Work out the finished part from the listing and answer in its coordinate system (mm). Face numbers are marked on the shaded views. A direction names the side the tool comes from. Give positions to 0.01 mm unless a question says otherwise; leave off trailing zeros. Loops run counter-clockwise (first coordinate to the right, second up) from the corner with the lowest first, then second, coordinate; pieces in that order, holes last. Notation, with made-up numbers: (74, 16.5) - (104, 16.5) arc R20 ccw to (104, 31.5) - close; hole circle Ø10 at (-1.75, -36). An arc over 180 degrees is marked (long way). One line per question, with ' | ' between items. Start each with the question number.
1. Find the intervals of material crossed by line 1 (Z direction, x = -7, y = 8.25); line 2 (Z direction, x = 7, y = 8.5); line 3 (Y direction, x = -20.4, z = 0), in increasing order.
2. Section B-B (y = 8.5) is taken. Determine the outline of the cut face in (x, z).
3. Each of these flat-tipped pins is pushed along its axis until it touches: pin 1 (3.5 mm diameter, centred on y = 8, z = 0, fed in from -X); pin 2 (4.5 mm diameter, centred on x = 0, y = -3, fed in from -Z); pin 3 (4 mm diameter, centred on y = -3, z = 0, fed in from +X). Where does it stop, or does it pass through?
4. For a pull along Z with two mould halves and no side action, classify the marked faces 4, 5 and 6 as released by +Z, released by -Z, zero draft, split by the parting line, or undercut.
5. Section A-A (y = -3) is taken. Give the number of separate pieces and of enclosed holes in the cut face, plus the area to 3 significant figures.
6. Which of the six approach directions +Z, -Z, +X, -X, +Y, -Y give full straight-line access (tool end or side, diameter ignored) to the marked faces 1, 2 and 3?
from build123d import *

# Parameters (mm, degrees)
SKETCH_1_R                = 19
SKETCH_1_R_2              = 1.45
SKETCH_1_R_3              = 2
EXTRUDE_1_DEPTH           = 12
SKETCH_2_R                = 1.45
SKETCH_2_R_2              = 2
EXTRUDE_2_DEPTH           = 7
SKETCH_3_R                = 1.45
CUT_EXTRUDE_1_DEPTH       = 48.5
SKETCH_4_R                = 1.45
CUT_EXTRUDE_2_DEPTH       = 48.5
SKETCH_5_R                = 1.45
CUT_EXTRUDE_3_DEPTH       = 39
SKETCH_8_R                = 24
CUT_EXTRUDE_6_DEPTH       = 5
SKETCH_10_R               = 24.25
EXTRUDE_3_DEPTH           = 3
SKETCH_11_R               = 21.9
EXTRUDE_4_DEPTH           = 18
CUT_EXTRUDE_7_DEPTH       = 18
SKETCH_13_R               = 1.45
CUT_EXTRUDE_8_DEPTH       = 43.25
CUT_EXTRUDE_8_DEPTH_BACK  = 7.25
SKETCH_14_R               = 1.45
CUT_EXTRUDE_9_DEPTH       = 53.294678888
CUT_EXTRUDE_9_DEPTH_BACK  = 17.294678888
SKETCH_15_R               = 1.45
CUT_EXTRUDE_10_DEPTH      = 43.25
CUT_EXTRUDE_10_DEPTH_BACK = 7.25
SKETCH_16_R               = 1.5
CUT_EXTRUDE_11_DEPTH      = 53.294678888
CUT_EXTRUDE_11_DEPTH_BACK = 17.294678888
FILLET_1_R                = 0.5
FILLET_2_R                = 2
SKETCH_17_R               = 1.45
SKETCH_17_R_2             = 2
SKETCH_17_R_3             = 2.272593427
EXTRUDE_5_DEPTH           = 9


with BuildPart() as part:
    # 草图1 → 凸台-拉伸1 (new body)
    with BuildSketch(Plane(origin=(0, 0, 0), x_dir=(1, 0, 0), z_dir=(0, 1, 0))):
        Circle(SKETCH_1_R)
        with Locations((0, 13.5)):
            Circle(SKETCH_1_R_2, mode=Mode.SUBTRACT)
        with Locations((-11.691342951, -6.75)):
            Circle(SKETCH_1_R_2, mode=Mode.SUBTRACT)
        with Locations((11.691342951, -6.75)):
            Circle(SKETCH_1_R_2, mode=Mode.SUBTRACT)
        with Locations((-10.522208656, 6.075)):
            Circle(SKETCH_1_R_3, mode=Mode.SUBTRACT)
        with Locations((0, -12.15)):
            Circle(SKETCH_1_R_3, mode=Mode.SUBTRACT)
        with Locations((10.522208656, 6.075)):
            Circle(SKETCH_1_R_3, mode=Mode.SUBTRACT)
    extrude(amount=EXTRUDE_1_DEPTH)

    # 草图2 → 凸台-拉伸2 (add)
    with BuildSketch(Plane(origin=(0, 12, 0), x_dir=(1, 0, 0), z_dir=(0, 1, 0))):
        Polygon((0, 21.939310229), (-19, 10.969655115), (-19, -10.969655115), (0, -21.939310229), (19, -10.969655115), (19, 10.969655115), align=None)
        with Locations((0, 13.5)):
            Circle(SKETCH_2_R, mode=Mode.SUBTRACT)
        with Locations((-10.522208656, 6.075)):
            Circle(SKETCH_2_R_2, mode=Mode.SUBTRACT)
        with Locations((10.522208656, 6.075)):
            Circle(SKETCH_2_R_2, mode=Mode.SUBTRACT)
        with Locations((-11.691342951, -6.75)):
            Circle(SKETCH_2_R, mode=Mode.SUBTRACT)
        with Locations((0, -12.15)):
            Circle(SKETCH_2_R_2, mode=Mode.SUBTRACT)
        with Locations((11.691342951, -6.75)):
            Circle(SKETCH_2_R, mode=Mode.SUBTRACT)
    extrude(amount=-EXTRUDE_2_DEPTH)

    # 草图3 → 切除-拉伸1 (cut, through all)
    with BuildSketch(Plane(origin=(9.5, 0, 16.454482672), x_dir=(0.866025404, 0, -0.5), z_dir=(0.5, 0, 0.866025404))):
        with Locations((0, 8.5)):
            Circle(SKETCH_3_R)
    extrude(amount=-CUT_EXTRUDE_1_DEPTH, mode=Mode.SUBTRACT)

    # 草图4 → 切除-拉伸2 (cut, through all)
    with BuildSketch(Plane(origin=(-9.5, 0, 16.454482672), x_dir=(0.866025404, 0, 0.5), z_dir=(-0.5, 0, 0.866025404))):
        with Locations((0, 8.5)):
            Circle(SKETCH_4_R)
    extrude(amount=-CUT_EXTRUDE_2_DEPTH, mode=Mode.SUBTRACT)

    # 草图5 → 切除-拉伸3 (cut, through all)
    with BuildSketch(Plane.ZY.offset(19)):
        with Locations((0, 8.5)):
            Circle(SKETCH_5_R)
    extrude(amount=-CUT_EXTRUDE_3_DEPTH, mode=Mode.SUBTRACT)

    # 草图8 → 切除-拉伸6 (cut)
    with BuildSketch(Plane.XZ):
        Circle(SKETCH_8_R)
    extrude(amount=-CUT_EXTRUDE_6_DEPTH, mode=Mode.SUBTRACT)

    # 草图10 → 凸台-拉伸3 (add)
    with BuildSketch(Plane.XZ.offset(-5)):
        Circle(SKETCH_10_R)
    extrude(amount=EXTRUDE_3_DEPTH)

    # 草图11 → 凸台-拉伸4 (add)
    with BuildSketch(Plane.XZ.offset(-2)):
        Circle(SKETCH_11_R)
    extrude(amount=EXTRUDE_4_DEPTH)

    # 草图12 → 切除-拉伸7 (cut)
    with BuildSketch(Plane.XZ.offset(16)):
        with BuildLine():
            Line((-15.656854249, -9.798989873), (-9.798989873, -15.656854249))
            ThreePointArc((-9.798989873, -15.656854249), (-7.203603083, -17.39103626), (-4.142135624, -18))
            Line((-4.142135624, -18), (4.142135624, -18))
            ThreePointArc((4.142135624, -18), (7.203603083, -17.39103626), (9.798989873, -15.656854249))
            Line((9.798989873, -15.656854249), (15.656854249, -9.798989873))
            ThreePointArc((15.656854249, -9.798989873), (17.39103626, -7.203603083), (18, -4.142135624))
            Line((18, -4.142135624), (18, 4.142135624))
            ThreePointArc((18, 4.142135624), (17.39103626, 7.203603083), (15.656854249, 9.798989873))
            Line((15.656854249, 9.798989873), (9.798989873, 15.656854249))
            ThreePointArc((9.798989873, 15.656854249), (7.203603083, 17.39103626), (4.142135624, 18))
            Line((4.142135624, 18), (-4.142135624, 18))
            ThreePointArc((-4.142135624, 18), (-7.203603083, 17.39103626), (-9.798989873, 15.656854249))
            Line((-9.798989873, 15.656854249), (-15.656854249, 9.798989873))
            ThreePointArc((-15.656854249, 9.798989873), (-17.39103626, 7.203603083), (-18, 4.142135624))
            Line((-18, 4.142135624), (-18, -4.142135624))
            ThreePointArc((-18, -4.142135624), (-17.39103626, -7.203603083), (-15.656854249, -9.798989873))
        make_face()
    extrude(amount=-CUT_EXTRUDE_7_DEPTH, mode=Mode.SUBTRACT)

    # 草图13 → 切除-拉伸8 (cut, two sides)
    with BuildSketch(Plane.ZY.offset(-18)) as cut_extrude_8_sk:
        with Locations((0, -3)):
            Circle(SKETCH_13_R)
    extrude(amount=CUT_EXTRUDE_8_DEPTH, mode=Mode.SUBTRACT)
    extrude(cut_extrude_8_sk.sketch, amount=-CUT_EXTRUDE_8_DEPTH_BACK, mode=Mode.SUBTRACT)

    # 草图14 → 切除-拉伸9 (cut, two sides)
    with BuildSketch(Plane(origin=(12.727922061, 0, -12.727922061), x_dir=(0.707106781, 0, 0.707106781), z_dir=(-0.707106781, 0, 0.707106781))) as cut_extrude_9_sk:
        with Locations((0, -11)):
            Circle(SKETCH_14_R)
    extrude(amount=CUT_EXTRUDE_9_DEPTH, mode=Mode.SUBTRACT)
    extrude(cut_extrude_9_sk.sketch, amount=-CUT_EXTRUDE_9_DEPTH_BACK, mode=Mode.SUBTRACT)

    # 草图15 → 切除-拉伸10 (cut, two sides)
    with BuildSketch(Plane.XY.offset(-18)) as cut_extrude_10_sk:
        with Locations((0, -3)):
            Circle(SKETCH_15_R)
    extrude(amount=CUT_EXTRUDE_10_DEPTH, mode=Mode.SUBTRACT)
    extrude(cut_extrude_10_sk.sketch, amount=-CUT_EXTRUDE_10_DEPTH_BACK, mode=Mode.SUBTRACT)

    # 草图16 → 切除-拉伸11 (cut, two sides)
    with BuildSketch(Plane(origin=(-12.727922061, 0, -12.727922061), x_dir=(0.707106781, 0, -0.707106781), z_dir=(0.707106781, 0, 0.707106781))) as cut_extrude_11_sk:
        with Locations((0, -11)):
            Circle(SKETCH_16_R)
    extrude(amount=CUT_EXTRUDE_11_DEPTH, mode=Mode.SUBTRACT)
    extrude(cut_extrude_11_sk.sketch, amount=-CUT_EXTRUDE_11_DEPTH_BACK, mode=Mode.SUBTRACT)

    # 圆角1
    fillet_1_edges = [part.edges().sort_by_distance(p)[0] for p in [
        (-21.9, -16, 0),
        (-7.203603083, -16, 17.39103626),
        (-12.727922061, -16, 12.727922061),
        (-17.39103626, -16, 7.203603083),
        (-18, -16, 0),
        (-17.39103626, -16, -7.203603083),
        (-12.727922061, -16, -12.727922061),
        (-7.203603083, -16, -17.39103626),
        (0, -16, -18),
        (7.203603083, -16, -17.39103626),
        (12.727922061, -16, -12.727922061),
        (17.39103626, -16, -7.203603083),
        (18, -16, 0),
        (17.39103626, -16, 7.203603083),
        (12.727922061, -16, 12.727922061),
        (7.203603083, -16, 17.39103626),
        (0, -16, 18),
    ]]
    fillet(fillet_1_edges, radius=FILLET_1_R)

    # 圆角2
    fillet_2_edges = [part.edges().sort_by_distance(p)[0] for p in [
        (-7.203603083, 2, 17.39103626),
        (0, 2, 18),
        (7.203603083, 2, 17.39103626),
        (12.727922061, 2, 12.727922061),
        (17.39103626, 2, 7.203603083),
        (18, 2, 0),
        (17.39103626, 2, -7.203603083),
        (12.727922061, 2, -12.727922061),
        (7.203603083, 2, -17.39103626),
        (0, 2, -18),
        (-7.203603083, 2, -17.39103626),
        (-12.727922061, 2, -12.727922061),
        (-17.39103626, 2, -7.203603083),
        (-18, 2, 0),
        (-17.39103626, 2, 7.203603083),
        (-12.727922061, 2, 12.727922061),
    ]]
    fillet(fillet_2_edges, radius=FILLET_2_R)

    # 草图17 → 凸台-拉伸5 (add)
    with BuildSketch(Plane(origin=(0, 12, 0), x_dir=(1, 0, 0), z_dir=(0, 1, 0))):
        with Locations((0, 13.5)):
            Circle(SKETCH_17_R)
        with Locations((10.522208656, 6.075)):
            Circle(SKETCH_17_R_2)
        with Locations((11.691342951, -6.75)):
            Circle(SKETCH_17_R)
        with Locations((0, -12.15)):
            Circle(SKETCH_17_R_2)
        with Locations((-11.691342951, -6.75)):
            Circle(SKETCH_17_R)
        with Locations((-10.522208656, 6.075)):
            Circle(SKETCH_17_R_3)
    extrude(amount=-EXTRUDE_5_DEPTH)


solid = part.part
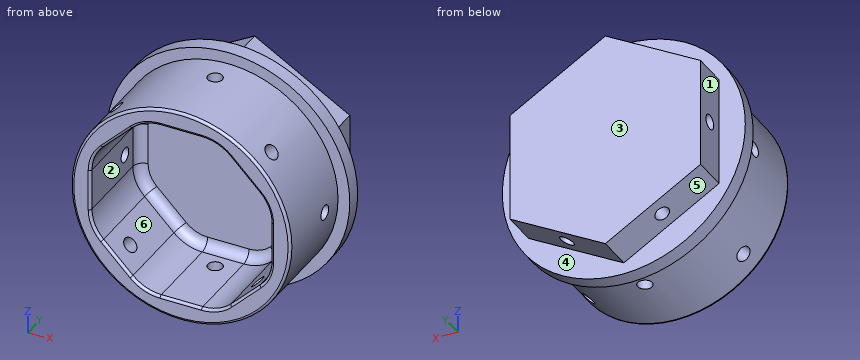
Conclusion:
1) line 1: -17.9 to -14.98, -9.27 to -1.43, 1.43 to 9.27, 14.98 to 17.9 | line 2: -17.9 to -15.02, -9.22 to -1.45, 1.45 to 9.22, 15.02 to 17.9 | line 3: -16 to -4.45, -1.55 to 5
2) outline: (-19, -10.97) - (-10.76, -15.73) - (-2.51, -1.45) - (-19, -1.45) - close; (-19, 1.45) - (-2.51, 1.45) - (-10.76, 15.73) - (-19, 10.97) - close; (-8.24, -17.18) - (0, -21.94) - (8.24, -17.18) - (0, -2.9) - close; (-8.24, 17.18) - (0, 2.9) - (8.24, 17.18) - (0, 21.94) - close; (2.51, -1.45) - (10.76, -15.73) - (19, -10.97) - (19, -1.45) - close; (2.51, 1.45) - (19, 1.45) - (19, 10.97) - (10.76, 15.73) - close
3) pin 1: x = -19 | pin 2: z = -21.9 | pin 3: x = 21.9
4) face 4: zero draft | face 5: released by -Z | face 6: undercut
5) separate pieces: 4 | enclosed holes: 0 | area: 399 mm²
6) face 1: +Z, -Z, -X, +Y | face 2: -Y | face 3: +Z, -Z, +X, -X, +Y
